Model file for the job. Use its own axes, mm. Face numbers are marked on the shaded views. A direction names the side the tool comes from. Round coordinates to 2 decimals unless told otherwise and drop trailing zeros. Loops run counter-clockwise (first coordinate to the right, second up) from the corner with the lowest first, then second, coordinate; pieces in that order, holes last. Notation, with made-up numbers: (47.5, 83.25) - (99.5, 83.25) arc R10 cw to (99.5, 102.25) - close; hole circle Ø5 at (0, -10). An arc over 180 degrees is marked (long way). Answer as a JSON object with one key per item and string values.
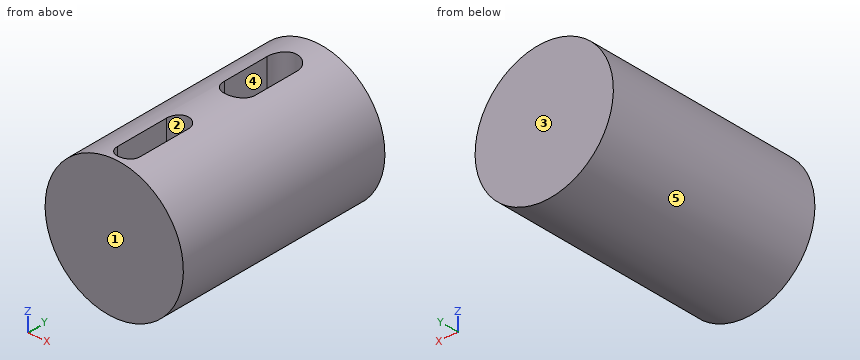
from build123d import *

# Parameters (mm, degrees)
SKETCH_1_R          = 40.061210901
EXTRUDE_1_DEPTH     = 130
CUT_EXTRUDE_1_DEPTH = 20


with BuildPart() as part:
    # 草图1 → 凸台-拉伸1 (new body)
    with BuildSketch(Plane(origin=(0, 0, 0), x_dir=(1, 0, 0), z_dir=(0, 1, 0))):
        with Locations(Location((0, 0, 0), (0, 0, 270))):
            Circle(SKETCH_1_R)
    extrude(amount=EXTRUDE_1_DEPTH)

    # 草图2 → 切除-拉伸1 (cut)
    with BuildSketch(Plane.XY.offset(40.061210901)):
        with BuildLine():
            Line((8.857338492, 108.295199344), (8.857338492, 81.062188459))
            ThreePointArc((8.857338492, 81.062188459), (0, 72.204849967), (-8.857338492, 81.062188459))
            Line((-8.857338492, 81.062188459), (-8.857338492, 108.295199344))
            ThreePointArc((-8.857338492, 108.295199344), (0, 117.152537836), (8.857338492, 108.295199344))
        make_face()
        with BuildLine():
            Line((6.477755016, 40.873667541), (6.477755016, 9.278086951))
            ThreePointArc((6.477755016, 9.278086951), (0, 2.800331935), (-6.477755016, 9.278086951))
            Line((-6.477755016, 9.278086951), (-6.477755016, 40.873667541))
            ThreePointArc((-6.477755016, 40.873667541), (0, 47.351422558), (6.477755016, 40.873667541))
        make_face()
    extrude(amount=-CUT_EXTRUDE_1_DEPTH, mode=Mode.SUBTRACT)


solid = part.part
1) Drop flat-ended pins along their axis: P1, Ø5.5, axis at y = 101, z = 28, coming from the -X side; P2, Ø12, axis at y = 44, z = 18.5, coming from the +X side; P3, Ø21.5, axis at y = 21.5, z = 27.5, coming from the -X side. Give the stop position or say it passes through.
Values follow:
{"P1": "x = -31.1", "P2": "x = 38.06", "P3": "x = -36.39"}
2) Slice it at D-D on z = 10.5. List the corners of the cut face in (x, y).
Values follow:
{"outline": "(-38.66, 0) - (38.66, 0) - (38.66, 130) - (-38.66, 130) - close"}
3) Probe probe 1 along Y at (x, z) = (3, 25); probe 2 along X at (y, z) = (25.5, 36.5); probe 3 along X at (y, z) = (45, 27.5). List the from-to ranges inside material, lowest first.
Values follow:
{"probe 1": "0 to 3.54, 46.61 to 72.73, 116.63 to 130", "probe 2": "-16.51 to -6.48, 6.48 to 16.51", "probe 3": "-29.13 to -4.99, 4.99 to 29.13"}
4) Tool access for the marked faces 1 and 2: list every direction of +Z, -Z, +X, -X, +Y, -Y with a clear straight run to the whole face (end or side of a thin tool).
Values follow:
{"face 1": "+Z, -Z, +X, -X, -Y", "face 2": "+Z"}
5) Slice it at A-A on z = 24. List the corners of the cut face in (x, y), then the cut area to 3 significant figures.
Values follow:
{"outline": "(-32.08, 0) - (32.08, 0) - (32.08, 130) - (-32.08, 130) - close; hole (-8.86, 81.06) arc R8.86 ccw to (8.86, 81.06) - (8.86, 108.3) arc R8.86 ccw to (-8.86, 108.3) - close; hole (-6.48, 9.28) arc R6.48 ccw to (6.48, 9.28) - (6.48, 40.87) arc R6.48 ccw to (-6.48, 40.87) - close", "area": "7,070 mm²"}
6) Slice it at C-C on y = 54. List the corners of the cut face in (x, z).
Values follow:
{"outline": "circle Ø80.12 at (0, 0)"}
7) Slice it at B-B on x = 0. List the corners of the cut face in (y, z), then the cut area to 3 significant figures.
Values follow:
{"outline": "(0, -40.06) - (130, -40.06) - (130, 40.06) - (117.15, 40.06) - (117.15, 20.06) - (72.2, 20.06) - (72.2, 40.06) - (47.35, 40.06) - (47.35, 20.06) - (2.8, 20.06) - (2.8, 40.06) - (0, 40.06) - close", "area": "8,630 mm²"}
8) Two-plate mould, pull along X, no slides. Class the marked faces 3, 4 and 5: pulls with the +X half, pulls with the -X half, needs draft (parallel to the pull), parting line crosses it, or undercut.
Values follow:
{"face 3": "needs draft", "face 4": "undercut", "face 5": "parting line crosses it"}
